Check sheet for the drawn part. Datum: minimum x, y, z corner. Units: mm. Give positions to 0.01 mm unless a question says otherwise; leave off trailing zeros. Write each loop counter-clockwise with the first axis right and the second up, starting at its lowest first coordinate (ties: lowest second). Pieces come first, ordered by that corner, then holes. Notation, with made-up numbers: (75, 21) - (107, 21) arc R22 cw to (107, 39) - close; hole circle Ø2 at (-18.75, -30). An arc over 180 degrees is marked (long way). Answer as a JSON object with one key per item and string values. Group by question number.
Item 1: Sectioned sample at D-D, the plane y = 2. Record the boundary of the cut face in (x, z), and give its area (3 significant figures).
Item 2: Sectioned sample at B-B, the plane z = 4.5. Record the boundary of the cut face in (x, y) (1 decimal).
Item 3: Sectioned sample at C-C, the plane y = 4.5. Record the boundary of the cut face in (x, z) (1 decimal).
Item 4: Scan lines: line 1 along Z through (x, y) = (17, 6.35) (1 decimal); line 2 along Y through (x, z) = (13, 10.75) (1 decimal); line 3 along Y through (x, z) = (16, 7.25). Record each from-to range of solid material in increasing order. Write a range as [from, to].
Item 5: Go/stop test with flat-tipped pins: pin 1 (2 mm diameter, centred on x = 14.5, z = 9, fed in from -Y); pin 2 (5 mm diameter, centred on x = 8.5, y = 4, fed in from -Z); pin 3 (3 mm diameter, centred on x = 11.5, y = 3.5, fed in from -Z). Record where each tip stops, or that it passes through.
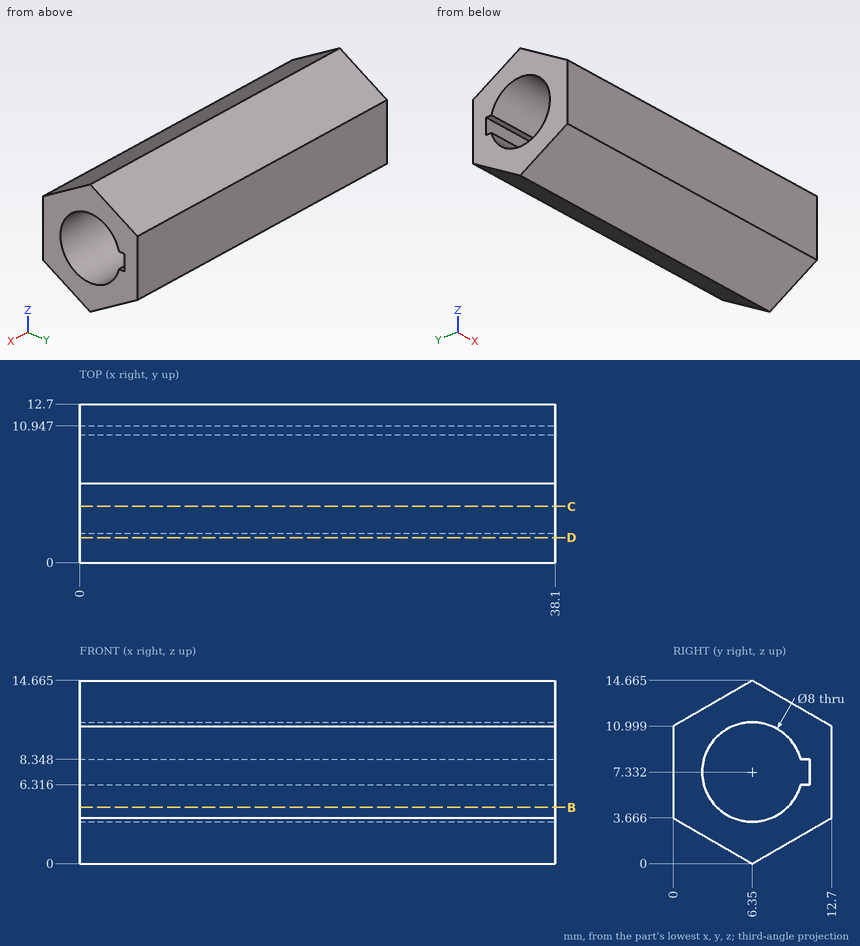
Geometry check:
{
 "1": {"outline": "(0, 2.51) - (38.1, 2.51) - (38.1, 12.15) - (0, 12.15) - close", "area": "367 mm^2"},
 "2": {"outline": "(0, 0) - (38.1, 0) - (38.1, 3.5) - (0, 3.5) - close; (0, 9.2) - (38.1, 9.2) - (38.1, 12.7) - (0, 12.7) - close"},
 "3": {"outline": "(0, 1.1) - (38.1, 1.1) - (38.1, 3.8) - (0, 3.8) - close; (0, 10.9) - (38.1, 10.9) - (38.1, 13.6) - (0, 13.6) - close"},
 "4": {"line 1": "[0, 3.3], [11.3, 14.7]", "line 2": "[0, 4.3], [8.4, 12.7]", "line 3": "[0, 2.35], [10.95, 12.7]"},
 "5": {"pin 1": "y = 0", "pin 2": "z = 0", "pin 3": "z = 0.78"}
}
